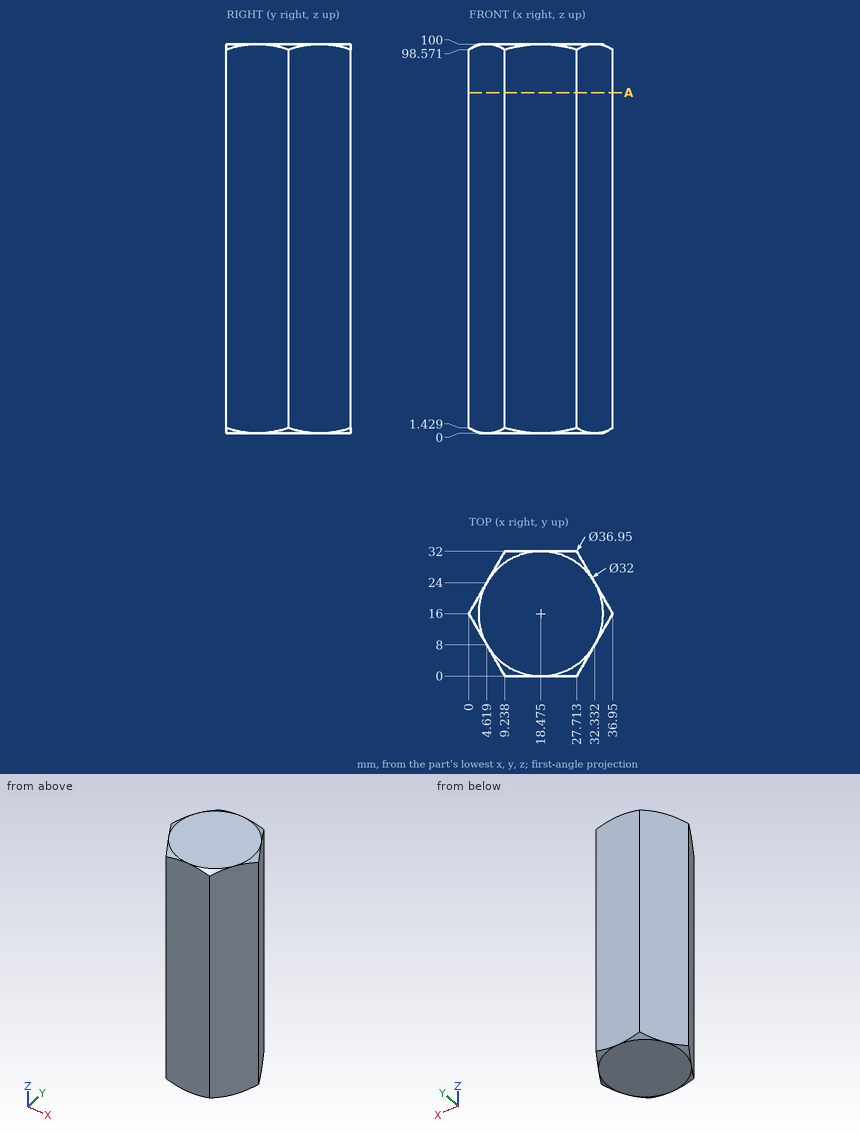
Could you check a few things on this drawing? It's one solid part, dimensions in mm from its lowest x, y, z. Round coordinates to 2 decimals unless told otherwise and drop trailing zeros. Loops run counter-clockwise (first coordinate to the right, second up) from the corner with the lowest first, then second, coordinate; pieces in that order, holes last. Notation, with made-up numbers: (73, -38.75) -> (109, -38.75) arc R6 cw to (109, -31.75) -> close; hole circle Ø11 at (43, 66). An arc over 180 degrees is marked (long way). One line per item, written item: value. Start each with the question number.
1. For pin 1 (4 mm diameter, centred on y = 19, z = 82, fed in from +X); pin 2 (12 mm diameter, centred on x = 33, z = 48, fed in from -Y); pin 3 (1 mm diameter, centred on x = 8.5, z = 82, fed in from -Y); pin 4 (4 mm diameter, centred on y = 26, z = 82.5, fed in from -X), each with a flat end and sliding along its axis, tell me the tip position at first contact or that it passes through.
2. If I drill on probe 1 along X at (y, z) = (4, 30.5); probe 2 along X at (y, z) = (2.5, 91) (1 decimal); probe 3 along Y at (x, z) = (28, 57) (1 decimal), over which ranges is the centre line in solid material (lowest first)?
3. If we section it at A-A, the plane z = 87.5: Write out the boundary of the cut face in (x, y), then the cut area to 3 significant figures.
Calculated:
1. pin 1: stops at x = 36.37
1. pin 2: stops at y = 0
1. pin 3: stops at y = 0.41
1. pin 4: stops at x = 4.62
2. probe 1: x = 6.93 to 30.02
2. probe 2: x = 7.8 to 29.2
2. probe 3: y = 0.5 to 31.5
3. outline: (0, 16) -> (9.24, 0) -> (27.71, 0) -> (36.95, 16) -> (27.71, 32) -> (9.24, 32) -> close
3. area: 887 mm²
